For this review, use the dimensioned drawing (mm, ordinates from the lowest corner) and the shaded views. Give positions to 0.01 mm unless a question says otherwise; leave off trailing zeros. Write each loop counter-clockwise with the first axis right and the second up, starting at its lowest first coordinate (ties: lowest second). Pieces come first, ordered by that corner, then holes. Notation, with made-up numbers: M 25,50 L 53,50 A24 cw 53,78 Z; hole C 34,77 d10. An arc over 180 degrees is marked long. One line per item, written item: value. Start each with the question number.
Item 1: Consider section D-D, the plane x = 64. Write out the cut boundary in (y, z).
Item 2: Mouldability with a two-part tool opening along X and no side actions: class the marked faces 1, 2, 3 and 4 as released by +X, released by -X, zero draft, split by the parting line, or undercut.
Item 3: To check wall thickness, follow probe 1 along Y at (x, z) = (35.45, 1.25); probe 2 along Y at (x, z) = (59.5, 0.8) (1 decimal); probe 3 along Y at (x, z) = (12.5, 1.5). State the ranges of each line that lie inside material, in increasing order.
Item 4: Consider section B-B, the plane x = 52.5. Write out the cut boundary in (y, z), and give its area (3 significant figures).
Item 5: Consider section C-C, the plane y = 35.45. Write out the cut boundary in (x, z).
Item 6: Clearance check with a flat-ended pin moving along its axis: pin 1 Ø1.5 at (x, y) = (48.5, 55) entering from +Z. State where the tip first meets the part, or that it passes through.
Item 7: Consider section A-A, the plane y = 14. Write out the cut boundary in (x, z).
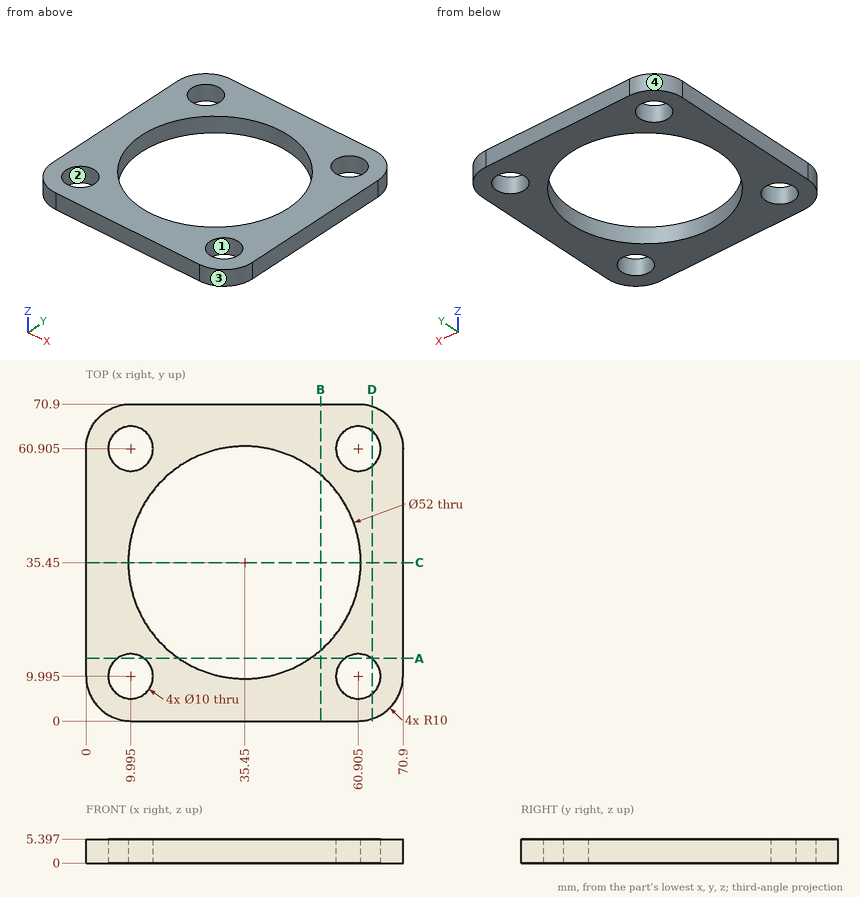
Model answer:
1. outline: M 0.49,0 L 6.07,0 L 6.07,5.4 L 0.49,5.4 Z; M 13.92,0 L 56.98,0 L 56.98,5.4 L 13.92,5.4 Z; M 64.83,0 L 70.41,0 L 70.41,5.4 L 64.83,5.4 Z
2. face 1: undercut
2. face 2: undercut
2. face 3: released by +X
2. face 4: released by -X
3. probe 1: y = 0 to 9.45, 61.45 to 70.9
3. probe 2: y = 0 to 5.2, 14.8 to 25.6, 45.3 to 56.1, 65.7 to 70.9
3. probe 3: y = 0 to 5.67, 14.32 to 23.23, 47.67 to 56.58, 65.23 to 70.9
4. outline: M 0,0 L 15.82,0 L 15.82,5.4 L 0,5.4 Z; M 55.08,0 L 70.9,0 L 70.9,5.4 L 55.08,5.4 Z
4. area: 171 mm2
5. outline: M 0,0 L 9.45,0 L 9.45,5.4 L 0,5.4 Z; M 61.45,0 L 70.9,0 L 70.9,5.4 L 61.45,5.4 Z
6. pin 1: passes through
7. outline: M 0,0 L 7,0 L 7,5.4 L 0,5.4 Z; M 12.99,0 L 20.76,0 L 20.76,5.4 L 12.99,5.4 Z; M 50.14,0 L 57.91,0 L 57.91,5.4 L 50.14,5.4 Z; M 63.9,0 L 70.9,0 L 70.9,5.4 L 63.9,5.4 Z
